Part print with two shaded views. Sizes in mm from the minimum x, y, z corner. A direction names the side the tool comes from. Coordinates: 2 decimals unless noted, no trailing zeros. Write each loop counter-clockwise with the first axis right and the second up, starting at its lowest first coordinate (ties: lowest second). Pieces come first, ordered by that corner, then holes.
Q1. Pin check, flat tips, straight feed: P1, Ø23.5, axis at x = 740, y = 40, coming from the +Z side; P2, Ø6.5, axis at x = 24.5, y = 94.5, coming from the +Z side; P3, Ø10, axis at x = 498, z = 25.5, coming from the -Y side; P4, Ø8, axis at x = 261, y = 13, coming from the +Z side. Stop position of each tip, or through.
Q2. Which spindle directions (+Z, -Z, +X, -X, +Y, -Y) get a long thin tool onto all of the face, cutting with end or side? Do the marked faces 1 and 2. Say none if no direction does.
Q3. Band-saw the part on C-C, the plane x = 316.5. Write the cut outline in (y, z), plus the area to 3 significant figures.
Q4. Band-saw the part on B-B, the plane z = 73. Write the cut outline in (x, y), plus the area to 3 significant figures.
Q5. Drill centre lines: probe 1 along Y at (x, z) = (40, 2.5); probe 2 along Y at (x, z) = (209, 13.5); probe 3 along Z at (x, y) = (201, 43). Where is each one in solid material? Low to high.
Q6. Band-saw the part on A-A, the plane y = 40. Write the cut outline in (x, z).
Q7. Band-saw the part on D-D, the plane y = 82.5. Write the cut outline in (x, z).
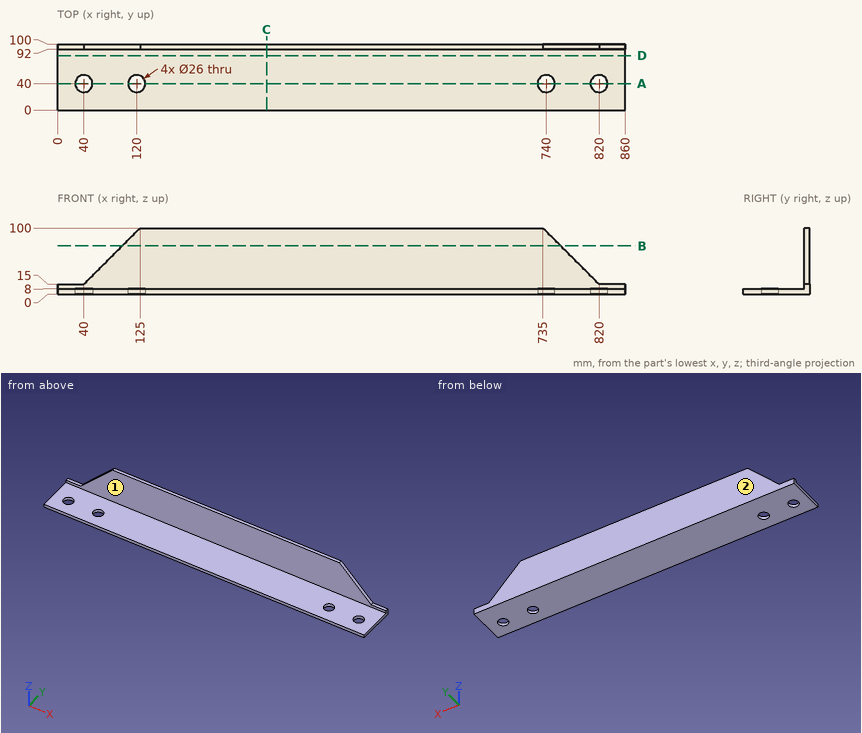
Answer sheet:
1. P1: passes through
1. P2: stops at z = 15
1. P3: stops at y = 92
1. P4: stops at z = 8
2. face 1: +Z, +X, -X, -Y
2. face 2: +Z, -Z, +X, -X, +Y
3. outline: (0, 0) - (100, 0) - (100, 100) - (92, 100) - (92, 8) - (0, 8) - close
3. area: 1,540 mm2
4. outline: (98, 92) - (762, 92) - (762, 100) - (98, 100) - close
4. area: 5,310 mm2
5. probe 1: y = 0 to 27, 53 to 100
5. probe 2: y = 92 to 100
5. probe 3: z = 0 to 8
6. outline: (0, 0) - (27, 0) - (27, 8) - (0, 8) - close; (53, 0) - (107, 0) - (107, 8) - (53, 8) - close; (133, 0) - (727, 0) - (727, 8) - (133, 8) - close; (753, 0) - (807, 0) - (807, 8) - (753, 8) - close; (833, 0) - (860, 0) - (860, 8) - (833, 8) - close
7. outline: (0, 0) - (860, 0) - (860, 8) - (0, 8) - close
